Part model, mm, in its own coordinate system. A direction names the side the tool comes from. Round coordinates to 2 decimals unless told otherwise and drop trailing zeros. Order: outer loops, then holes, each group sorted by start corner. A loop starts at its lowest first (then second) coordinate and runs counter-clockwise, first axis right, second up. Notation, with made-up numbers: (-20.75, 51.5) - (-16.75, 51.5) arc R9 ccw to (-16.75, 55.5) - close; hole circle Ø4 at (-7.5, 44). An arc over 180 degrees is marked (long way). Answer as a JSON object with one key per item and string values.
```python
from build123d import *

# Parameters (mm, degrees)
F1_DEPTH = 2000


with BuildPart() as f1:
    # F0 (on Top) → F1 (new body)
    with BuildSketch(Plane.XY):
        with BuildLine():
            Line((140, 1), (0, 1))
            Line((0, 1), (-140, 1))
            ThreePointArc((-140, 1), (-140.865758, 0.905184), (-141.690473, 0.625231))
            Line((-141.690473, 0.625231), (-232.321252, -41.636595))
            Line((-232.321252, -41.636595), (-231.476015, -43.449211))
            Line((-231.476015, -43.449211), (-140.845237, -1.187384))
            ThreePointArc((-140.845237, -1.187384), (-140.432879, -1.047408), (-140, -1))
            Line((-140, -1), (0, -1))
            Line((0, -1), (140, -1))
            ThreePointArc((140, -1), (140.432879, -1.047408), (140.845237, -1.187384))
            Line((140.845237, -1.187384), (231.476015, -43.449211))
            Line((231.476015, -43.449211), (232.321252, -41.636595))
            Line((232.321252, -41.636595), (141.690473, 0.625231))
            ThreePointArc((141.690473, 0.625231), (140.865758, 0.905184), (140, 1))
        make_face()
    extrude(amount=F1_DEPTH)


solid = f1.part
```
Item 1: Tool access for faces 4 (the flat face through (187.64, -20.8, 986)), 5 (the flat face through (185.526, -22.022, 986)): list every direction of +Z, -Z, +X, -X, +Y, -Y with a clear straight run to the whole face (end or side of a thin tool).
Taken from the geometry:
{"face 4": "+Z, -Z, +X, +Y", "face 5": "+Z, -Z, -Y"}
Item 2: Two-plate mould, pull along X, no slides. Class faces 1 (the flat face through (-186.37, -20.21, 986)), 2 (the flat face through (2, 1, 986)), 3 (the flat face through (-186.795, -22.614, 986)): pulls with the +X half, pulls with the -X half, needs draft (parallel to the pull), parting line crosses it, or undercut.
Taken from the geometry:
{"face 1": "pulls with the -X half", "face 2": "needs draft", "face 3": "undercut"}
Item 3: Cut at D-D (x = -192.5). Write the cut outline in (y, z), plus the area to 3 significant figures.
Taken from the geometry:
{"outline": "(-25.27, 0) - (-23.07, 0) - (-23.07, 2000) - (-25.27, 2000) - close", "area": "4,410 mm2"}
Item 4: Cut at B-B (z = 995). Write the cut outline in (x, y), plus the area to 3 significant figures.
Taken from the geometry:
{"outline": "(-232.32, -41.64) - (-231.48, -43.45) - (-140.85, -1.19) arc R2 cw to (-140, -1) - (140, -1) arc R2 cw to (140.85, -1.19) - (231.48, -43.45) - (232.32, -41.64) - (141.69, 0.63) arc R4 ccw to (140, 1) - (-140, 1) arc R4 ccw to (-141.69, 0.63) - close", "area": "965 mm2"}
Item 5: Cut at A-A (y = -21). Write the cut outline in (x, z).
Taken from the geometry:
{"outline": "(-188.07, 0) - (-183.33, 0) - (-183.33, 2000) - (-188.07, 2000) - close; (183.33, 0) - (188.07, 0) - (188.07, 2000) - (183.33, 2000) - close"}
Item 6: Drop flat-ended pins along their axis: P1, Ø1, axis at y = -22, z = 428, coming from the -X side; P2, Ø2, axis at y = -11.5, z = 260, coming from the +X side; P3, Ø8, axis at y = -25.5, z = 1270.5, coming from the +X side. Give the stop position or say it passes through.
Taken from the geometry:
{"P1": "x = -191.28", "P2": "x = 169.84", "P3": "x = 206.29"}
Item 7: Cut at C-C (x = 36). Write the cut outline in (y, z).
Taken from the geometry:
{"outline": "(-1, 0) - (1, 0) - (1, 2000) - (-1, 2000) - close"}
Item 8: Probe L1, parallel to Y at x = 25, z = 1864.5; L2, parallel to X at y = -24, z = 159.5; L3, parallel to X at y = -40.5, z = 1865. List the from-to ranges inside material, lowest first. Write a range as from..to.
Taken from the geometry:
{"L1": "-1..1", "L2": "-194.5..-189.77, 189.77..194.5", "L3": "-229.88..-225.15, 225.15..229.88"}
